Could you check a few things on this model? Use its own coordinates, in mm. A direction names the side the tool comes from. Coordinates: 2 decimals unless noted, no trailing zeros. Loops run counter-clockwise (first coordinate to the right, second up) from the corner with the lowest first, then second, coordinate; pieces in that order, holes last. Notation, with made-up numbers: (-6, 16.5) - (16, 16.5) arc R20 cw to (16, 46.5) - close; hole circle Ø1 at (28.5, 21). An arc over 180 degrees is marked (long way). Use CSV: the item, a comma, the result in double quotes.
from build123d import *

# Parameters (mm, degrees)
EXTRUDE_1_DEPTH     = 17.5
SKETCH_3_W          = 24
SKETCH_3_H          = 9
SKETCH_3_R          = 3.5
CUT_EXTRUDE_1_DEPTH = 4
SKETCH_6_R          = 4
CUT_EXTRUDE_2_DEPTH = 9.05
SKETCH_7_R          = 4
CUT_EXTRUDE_3_DEPTH = 4.75
SKETCH_8_R          = 1.616666667
CUT_EXTRUDE_4_DEPTH = 38.428601697
FILLET_1_R          = 0.5
EXTRUDE_START       = -1
SKETCH_9_R          = 3.5
SKETCH_9_R_2        = 0.75
EXTRUDE_2_DEPTH     = 1


with BuildPart() as part:
    # Эскиз1 → Бобышка-Вытянуть1 (new, symmetric)
    with BuildSketch(Plane(origin=(0, 0, 0), x_dir=(0, 0, -1), z_dir=(1, 0, 0))):
        with BuildLine():
            Line((-7.765, 7), (7.765, 7))
            ThreePointArc((7.765, 7), (11.265, 3.5), (7.765, 0))
            Line((7.765, 0), (-7.765, 0))
            ThreePointArc((-7.765, 0), (-11.265, 3.5), (-7.765, 7))
        make_face()
    extrude(amount=EXTRUDE_1_DEPTH, both=True)

    # Эскиз3 → Вырез-Вытянуть1 (cut)
    with BuildSketch(Plane(origin=(17.5, 0, 0), x_dir=(0, 0, -1), z_dir=(1, 0, 0))):
        with Locations((0, 3.5)):
            Rectangle(SKETCH_3_W, SKETCH_3_H)
        with Locations(Location((-7.765, 3.5, 0), (0, 0, 90))):
            Circle(SKETCH_3_R, mode=Mode.SUBTRACT)
    cut_extrude_1 = extrude(amount=-CUT_EXTRUDE_1_DEPTH, mode=Mode.SUBTRACT)

    # Зеркальное отражение1: Вырез-Вытянуть1 across plane
    add(cut_extrude_1.mirror(Plane(origin=(0, 0, 0), x_dir=(0, 0, 1), z_dir=(1, 0, 0))), mode=Mode.SUBTRACT)

    # Эскиз6 → Вырез-Вытянуть2 (cut, symmetric)
    with BuildSketch(Plane(origin=(0, 0, 0), x_dir=(0, 0, -1), z_dir=(1, 0, 0))):
        with Locations((-7.765, 3.5)):
            Circle(SKETCH_6_R)
    extrude(amount=CUT_EXTRUDE_2_DEPTH, both=True, mode=Mode.SUBTRACT)

    # Эскиз7 → Вырез-Вытянуть3 (cut)
    with BuildSketch(Plane(origin=(13.5, 0, 0), x_dir=(0, 0, -1), z_dir=(1, 0, 0))):
        with Locations((7.765, 3.5)):
            Circle(SKETCH_7_R)
    cut_extrude_3 = extrude(amount=-CUT_EXTRUDE_3_DEPTH, mode=Mode.SUBTRACT)

    # Зеркальное отражение2: Вырез-Вытянуть3 across plane
    add(cut_extrude_3.mirror(Plane(origin=(0, 0, 0), x_dir=(0, 0, 1), z_dir=(1, 0, 0))), mode=Mode.SUBTRACT)

    # Эскиз8 → Вырез-Вытянуть4 (cut, through all)
    with BuildSketch(Plane(origin=(17.5, 0, 0), x_dir=(0, 0, -1), z_dir=(1, 0, 0))):
        with Locations((7.765, 3.5)):
            Circle(SKETCH_8_R)
        Polygon((-9.035170592, 2.766666667), (-7.765, 4.966666667), (-6.494829408, 2.766666667), align=None)
    extrude(amount=-CUT_EXTRUDE_4_DEPTH, mode=Mode.SUBTRACT)

    # Скругление1
    fillet_1_edges = [part.edges().sort_by_distance(p)[0] for p in [
        (0, 7, 5.828508327),
        (0, 0, 5.828508327),
        (11.125, 0, -5.828508327),
        (11.125, 7, -5.828508327),
        (-11.125, 0, -5.828508327),
        (-11.125, 7, -5.828508327),
    ]]
    fillet(fillet_1_edges, radius=FILLET_1_R)

    # Эскиз9 → Бобышка-Вытянуть2 (add)
    with BuildSketch(Plane.ZY.offset(17.5).offset(EXTRUDE_START)):
        with Locations(Location((7.765, 3.5, 0), (0, 0, 90))):
            Circle(SKETCH_9_R)
        with Locations((7.765, 3.5)):
            Circle(SKETCH_9_R_2, mode=Mode.SUBTRACT)
    extrude(amount=EXTRUDE_2_DEPTH)


solid = part.part
(1) Suppose I cut it at B-B (x = 3). Write out the boundary of the cut face in (y, z) (3 decimals), plus the area to 3 significant figures.
Computed:
outline,"(0, -7.765) arc R3.5 ccw to (7, -7.765) - (7, 4.411) arc R0.5 ccw to (6.167, 4.784) arc R4 cw to (0.833, 4.784) arc R0.5 ccw to (0, 4.411) - close; hole circle Ø3.233 at (3.5, -7.765)"
area,"95.2 mm²"
(2) Suppose I cut it at C-C (y = 1.25). Write out the boundary of the cut face in (x, z).
Computed:
outline,"(-17.5, 5.08) - (-13.5, 5.08) - (-13.5, -4.46) - (-8.75, -4.46) - (-8.75, -10.45) - (8.75, -10.45) - (8.75, -4.46) - (13.5, -4.46) - (13.5, 5.08) - (17.5, 5.08) - (17.5, 10.45) - (9.05, 10.45) - (9.05, 4.46) - (-9.05, 4.46) - (-9.05, 10.45) - (-17.5, 10.45) - close"
(3) Suppose I cut it at D-D (x = 13). Write out the boundary of the cut face in (y, z) (3 decimals), plus the area to 3 significant figures.
Computed:
outline,"(0, -4.411) arc R0.5 ccw to (0.833, -4.784) arc R4 cw to (6.167, -4.784) arc R0.5 ccw to (7, -4.411) - (7, 7.765) arc R3.5 ccw to (0, 7.765) - close; hole (2.767, 6.495) - (4.967, 7.765) - (2.767, 9.035) - close"
area,"101 mm²"
(4) Which directions (+Z, -Z, +X, -X, +Y, -Y) give clear straight access to the entire face, cutting with the end or side of a thin tool? Please do faces 4 (the face through (-16.993, 3.133, 7.111)), 5 (the face through (0.127, 6.711, 4.864)), 6 (the face through (11.158, 0.289, -4.864)).
Computed:
face 4,"+X, -X"
face 5,"+Z"
face 6,"-Z, +X"
(5) Please list where these lines run through material, in increasing order: line 1 (X direction, y = 2.25, z = 10); line 2 (X direction, y = 1.5, z = -9.5); line 3 (X direction, y = 1.5, z = 4.25).
Computed:
line 1,"x = -17.5 to -9.05, 9.05 to 17.5"
line 2,"x = -8.75 to 8.75"
line 3,"x = -13.5 to 13.5"
(6) Thinking about a two-plate mould opening in Y: for faces 1 (the face through (-17.5, 4, 7)), 2 (the face through (0, 7, 0)), 3 (the face through (-16.5, 4.4, 7.8)), which applies, +Y half, -Y half, draft (parallel to the pull), parting line (faces both ways), or undercut?
Computed:
face 1,"draft"
face 2,"+Y half"
face 3,"undercut"
(7) Suppose I cut it at A-A (z = 9.5). Write out the boundary of the cut face in (x, y), plus the area to 3 significant figures.
Computed:
outline,"(-17.5, 0.46) - (-9.05, 0.46) - (-9.05, 6.54) - (-17.5, 6.54) - close; (9.05, 0.46) - (17.5, 0.46) - (17.5, 6.54) - (9.05, 6.54) - close"
area,"103 mm²"
(8) Will these pins go through, and if not, where does the flat tip stop? pin 1 (2 mm diameter, centred on y = 3, z = -1, fed in from +X); pin 2 (1.5 mm diameter, centred on y = 3.5, z = -5.5, fed in from -X); pin 3 (3.5 mm diameter, centred on y = 3.5, z = -1, fed in from -X).
Computed:
pin 1,"stops at x = 13.5"
pin 2,"stops at x = -8.75"
pin 3,"stops at x = -13.5"
